```python
from build123d import *

# Parameters (mm, degrees)
PAD001_DEPTH = 29
SKETCH001_R  = 5.955
PAD_DEPTH    = 51.001
PAD002_DEPTH = 11
PAD003_DEPTH = 13


with BuildPart() as body:
    # Sketch → Pad001 (new body)
    with BuildSketch(Plane.XY):
        with BuildLine():
            ThreePointArc((-1.5, 5.762988), (0, -5.955), (1.5, 5.762988))
            Line((1.5, 3.762988), (1.5, 5.762988))
            Line((-1.5, 3.762988), (1.5, 3.762988))
            Line((-1.5, 5.762988), (-1.5, 3.762988))
        make_face()
    extrude(amount=PAD001_DEPTH)


with BuildPart() as body_1:
    # Body placement: moved
    add(body.part.moved(Location((0, 0, 51))))


with BuildPart() as shifter_shaft:
    # Sketch001 → Pad (new body)
    with BuildSketch(Plane.XY):
        Circle(SKETCH001_R)
    extrude(amount=PAD_DEPTH)

    # Fusion: union Body
    add(body_1.part)


with BuildPart() as body003:
    # Sketch003 → Revolution (revolve)
    with BuildSketch(Plane.XY):
        Polygon((-3, 1.5), (-3, 4.5), (-11.91, 4.5), (-11.91, 0), (11.91, 0), (11.91, 4.5), (3, 4.5), (3, 1.5), align=None)
    revolve(axis=Axis((0, 0, 0), (1, 0, 0)))


with BuildPart() as body003_1:
    # Body003 placement: moved
    add(body003.part.moved(Location((0, 9.455, 5.5))))


with BuildPart() as cut:
    # Sketch002 → Pad002 (new body)
    with BuildSketch(Plane.XY):
        with BuildLine():
            ThreePointArc((-1.712437, 5.703471), (0, -5.955), (1.712437, 5.703471))
            ThreePointArc((1, 6.661233), (1.19764, 6.064393), (1.712437, 5.703471))
            Line((1, 6.661233), (1, 12.21))
            ThreePointArc((1.7, 12.91), (1.205025, 12.704975), (1, 12.21))
            Line((4.32426, 12.91), (1.7, 12.91))
            ThreePointArc((5.252076, 12.283038), (4.884154, 12.738564), (4.32426, 12.91))
            Line((8.772501, 3.527074), (5.252076, 12.283038))
            ThreePointArc((-8.772501, 3.527074), (0, -9.455), (8.772501, 3.527074))
            Line((-8.772501, 3.527074), (-5.252076, 12.283038))
            ThreePointArc((-4.32426, 12.91), (-4.884154, 12.738564), (-5.252076, 12.283038))
            Line((-4.32426, 12.91), (-1.7, 12.91))
            ThreePointArc((-1, 12.21), (-1.205025, 12.704975), (-1.7, 12.91))
            Line((-1, 6.661233), (-1, 12.21))
            ThreePointArc((-1.712437, 5.703471), (-1.19764, 6.064393), (-1, 6.661233))
        make_face()
    extrude(amount=PAD002_DEPTH)

    # Sketch004 (on Face16 of Pad002) → Pad003 (join)
    with BuildSketch(Plane.XY.offset(11)):
        with BuildLine():
            ThreePointArc((-1.712437, 5.703471), (0, -5.955), (1.712437, 5.703471))
            ThreePointArc((1, 6.661233), (1.19764, 6.064393), (1.712437, 5.703471))
            Line((1, 6.661233), (1, 8.215049))
            ThreePointArc((2.236546, 9.186669), (1.38216, 9.001352), (1, 8.215049))
            ThreePointArc((-2.236546, 9.186669), (0, -9.455), (2.236546, 9.186669))
            ThreePointArc((-1, 8.215049), (-1.38216, 9.001352), (-2.236546, 9.186669))
            Line((-1, 6.661233), (-1, 8.215049))
            ThreePointArc((-1.712437, 5.703471), (-1.19764, 6.064393), (-1, 6.661233))
        make_face()
    extrude(amount=PAD003_DEPTH)

    # Cut: cut Body003
    add(body003_1.part, mode=Mode.SUBTRACT)


with BuildPart() as cut001:
    # Sphere → Sphere (revolve)
    with BuildSketch(Plane(origin=(0, 0, 52), x_dir=(1, 0, 0), z_dir=(0, -1, 0))):
        with BuildLine():
            ThreePointArc((0, -31), (31, 0), (0, 31))
            Line((0, 31), (0, -31))
        make_face()
    revolve(axis=Axis((0, 0, 52), (0, 0, 1)))

    # Fusion001: union Cut
    add(cut.part)

    # Cut001: cut Shifter_shaft
    add(shifter_shaft.part, mode=Mode.SUBTRACT)


solid = cut001.part
```
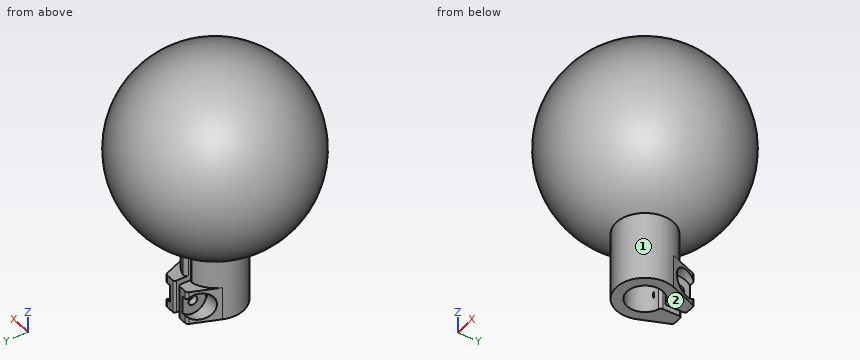
Geometry: final body of the model. Coordinates: model frame, mm. Face numbers are marked on the shaded views. Round coordinates to 2 decimals unless told otherwise and drop trailing zeros. Order: outer loops, then holes, each group sorted by start corner. A loop starts at its lowest first (then second) coordinate and runs counter-clockwise, first axis right, second up. Notation, with made-up numbers: M 48.5,61 L 90.5,61 A24 ccw 90.5,89 Z; hole C 10.5,66 d9. An arc over 180 degrees is marked long. One line per item, written item: value.
(1) Cut plane A-A (y = 0). Return the cut outline in (x, z) (3 decimals).
Result sheet:
outline: M -9.455,0 L -5.955,0 L -5.955,80 L 5.955,80 L 5.955,0 L 9.455,0 L 9.455,22.477 A31 ccw long -9.455,22.477 Z
(2) Line query: probe 1 along X at (y, z) = (5, 70); probe 2 along Z at (x, y) = (-4, 11.5); probe 3 along X at (y, z) = (-3, 39). Output: solid intervals per line, ascending. Write a range as [from, to].
Result sheet:
probe 1: [-24.74, -3.23], [-1.5, 1.5], [3.23, 24.74]
probe 2: [0, 1.49], [9.51, 11], [23.49, 80.51]
probe 3: [-27.98, -5.14], [5.14, 27.98]
(3) Cut plane D-D (z = 62.5). Return the cut outline in (x, y) (3 decimals), and give its area (3 significant figures).
Result sheet:
outline: C 0,0 d58.335; hole M -1.5,3.763 L -1.5,5.763 A5.955 ccw long 1.5,5.763 L 1.5,3.763 Z
area: 2,570 mm2
(4) Cut plane C-C (x = 0). Return the cut outline in (y, z) (3 decimals).
Result sheet:
outline: M -9.455,0 L -5.955,0 L -5.955,80 L 3.763,80 L 3.763,51.001 L 5.955,51.001 L 5.955,21.577 A31 ccw long -9.455,22.477 Z
(5) Pin query (flat end, axial travel): P1, Ø4.5, axis at y = 10, z = 7.5, coming from the +X side; P2, Ø11.5, axis at y = 9.455, z = 5.5, coming from the +X side; P3, Ø1.3, axis at x = -3, z = 3, coming from the +Y side. Return the tip coordinate at first contact, or that it passes through.
Result sheet:
P1: x = 3
P2: x = 8.7
P3: y = 12.91
(6) Cut plane B-B (z = 5.5). Return the cut outline in (x, y) (1 decimal).
Result sheet:
outline: M -8.8,3.5 A9.5 ccw long 8.8,3.5 L 8.2,5 L 3.3,5 A6 cw long -3.3,5 L -8.2,5 Z; M -3,5.1 A6 cw -1.7,5.7 A1 ccw -1,6.7 L -1,8 L -3,8 Z; M -3,11 L -1,11 L -1,12.2 A0.7 ccw -1.7,12.9 L -3,12.9 Z; M 1,6.7 A1 ccw 1.7,5.7 A6 cw 3,5.1 L 3,8 L 1,8 Z; M 1,11 L 3,11 L 3,12.9 L 1.7,12.9 A0.7 ccw 1,12.2 Z
(7) Pull-direction query (Z, two-part tool) for the marked faces 1 and 2; classes: pulls with the +Z half, pulls with the -Z half, needs draft (parallel to the pull), parting line crosses it, or undercut.
Result sheet:
face 1: undercut
face 2: pulls with the -Z half
